Design review of the part built by this model. Coordinates are the model's own, in mm. Face numbers are marked on the shaded views. A direction names the side the tool comes from. Round coordinates to 2 decimals unless told otherwise and drop trailing zeros. Order: outer loops, then holes, each group sorted by start corner. A loop starts at its lowest first (then second) coordinate and runs counter-clockwise, first axis right, second up.
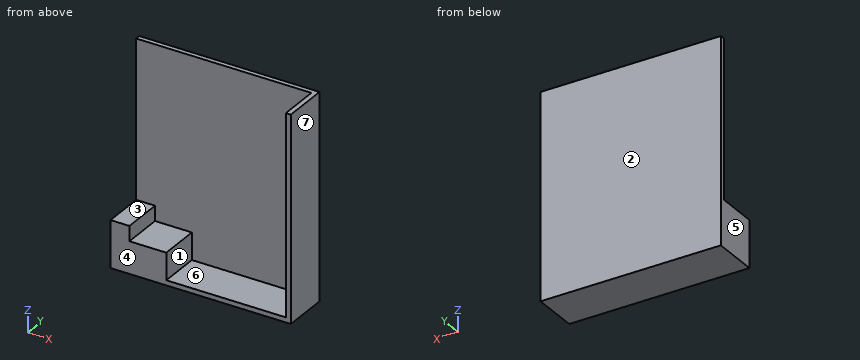
from build123d import *

# Parameters (mm, degrees)
F0_W     = 370
F0_H     = 270
F0_W_2   = 50
F0_H_2   = 2000
F1_DEPTH = 410
F2_W     = 1810
F2_H     = 2050
F3_DEPTH = 50


with BuildPart() as f1:
    # F0 (on Front) → F1 (new body)
    with BuildSketch(Plane.XZ):
        Polygon((-1853.846294, 0), (-2223.846294, 0), (-2413.846294, 0), (-2413.846294, -50), (-603.846294, -50), (-603.846294, 0), (-653.846294, 0), align=None)
        Polygon((-2413.846294, 0), (-2223.846294, 0), (-2223.846294, 270), (-2223.846294, 420), (-2413.846294, 420), align=None)
        with Locations((-2038.846294, 135)):
            Rectangle(F0_W, F0_H)
        with Locations((-628.846294, 1000)):
            Rectangle(F0_W_2, F0_H_2)
    extrude(amount=F1_DEPTH)

    # F2 (on face) → F3 (join)
    with BuildSketch(Plane(origin=(0, 0, 0), x_dir=(-1, 0, 0), z_dir=(0, 1, 0))):
        with Locations((1508.846294, 975)):
            Rectangle(F2_W, F2_H)
    extrude(amount=F3_DEPTH)


solid = f1.part
1) Clearance check with flat-ended pins moving along their axes: P1, Ø3, axis at x = -914.5, y = -249.5, coming from the +Z side; P2, Ø1, axis at x = -1978.5, y = -162.5, coming from the +Z side; P3, Ø5, axis at x = -1246, z = 1536, coming from the -Y side. State where each tip first meets the part, or that it passes through.
Results:
P1: stops at z = 0
P2: stops at z = 270
P3: stops at y = 0
2) Take a section at B-B on z = 394.5. Give the boundary of the cut face in (x, y).
Results:
outline: (-2413.85, -410) - (-2223.85, -410) - (-2223.85, 0) - (-653.85, 0) - (-653.85, -410) - (-603.85, -410) - (-603.85, 50) - (-2413.85, 50) - close
3) To check wall thickness, follow line 1 along X through (y, z) = (-249.5, 61.5); line 2 along Z through (x, y) = (-2151.5, -73); line 3 along Y through (x, z) = (-1157.5, 1830). State the ranges of each line that lie inside material, in increasing order.
Results:
line 1: x = -2413.85 to -1853.85, -653.85 to -603.85
line 2: z = -50 to 270
line 3: y = 0 to 50
4) Take a section at A-A on y = -325.5. Give the boundary of the cut face in (x, z), plus the area to 3 significant figures.
Results:
outline: (-2413.85, -50) - (-603.85, -50) - (-603.85, 2000) - (-653.85, 2000) - (-653.85, 0) - (-1853.85, 0) - (-1853.85, 270) - (-2223.85, 270) - (-2223.85, 420) - (-2413.85, 420) - close
area: 370,000 mm2
5) The part is to be moulded in two halves that separate along X. For the marked faces 4, 5, 6 and 7, say which applies: released by +X, released by -X, zero draft, split by the parting line, or undercut.
Results:
face 4: zero draft
face 5: released by -X
face 6: undercut
face 7: released by +X
6) Take a section at D-D on z = 1618.5. Give the boundary of the cut face in (x, y), plus the area to 3 significant figures.
Results:
outline: (-2413.85, 0) - (-653.85, 0) - (-653.85, -410) - (-603.85, -410) - (-603.85, 50) - (-2413.85, 50) - close
area: 111,000 mm2
7) Take a section at C-C on x = -788.5. Give the boundary of the cut face in (y, z), plus the area to 3 significant figures.
Results:
outline: (-410, -50) - (50, -50) - (50, 2000) - (0, 2000) - (0, 0) - (-410, 0) - close
area: 123,000 mm2
8) For the marked faces 1, 2 and 3, list the 3-axis set-ups (+Z, -Z, +X, -X, +Y, -Y) from which the entire face can be reached by the end or side of a thin tool; tool diameter is ignored.
Results:
face 1: +Z, -Y
face 2: +Z, -Z, +X, -X, +Y
face 3: +Z, -X, -Y
